from build123d import *

# Parameters (mm, degrees)
F4_R      = 3.75
F4_R_2    = 2
F9_DEPTH  = 1.2
F10_DEPTH = 3.7
F11_DEPTH = 3
F12_DEPTH = 2.5
F13_DEPTH = 8
F14_D     = 2.5
F14_DEPTH = 6.0511758158
F15_D     = 1.4
F15_DEPTH = 11.001


with BuildPart() as f8:
    # F3 (on Front) → F8 (revolve)
    with BuildSketch(Plane.XZ):
        with BuildLine():
            Line((0, 42.7), (0, 0))
            Line((0, 0), (-8.38e-08, -21.7723533995))
            Line((-8.38e-08, -21.7723533995), (0.7499999162, -21.7723533995))
            Line((0.7499999162, -21.7723533995), (1.9999999162, -19))
            Line((1.9999999162, -19), (1.9999999162, -1.2))
            Line((1.9999999162, -1.2), (3.7499999162, -1.2))
            Line((3.7499999162, -1.2), (3.7499999162, 0))
            Line((3.7499999162, 0), (11, 0))
            Line((11, 0), (11, 1.6))
            Line((11, 1.6), (4.5, 1.6))
            Line((4.5, 1.6), (4.5, 2.6))
            Line((4.5, 2.6), (11, 2.6))
            Line((11, 2.6), (11, 4.1))
            Line((11, 4.1), (4.5, 4.1))
            Line((4.5, 4.1), (4.5, 5.1))
            Line((4.5, 5.1), (11, 5.1))
            Line((11, 5.1), (11, 6.6))
            Line((11, 6.6), (4.5, 6.6))
            Line((4.5, 6.6), (4.5, 7.6))
            Line((4.5, 7.6), (11, 7.6))
            Line((11, 7.6), (11, 9.1))
            Line((11, 9.1), (4.5, 9.1))
            Line((4.5, 9.1), (4.5, 10.1))
            Line((4.5, 10.1), (11, 10.1))
            Line((11, 10.1), (11, 11.6))
            Line((11, 11.6), (4.5, 11.6))
            Line((4.5, 11.6), (4.5, 12.6))
            Line((4.5, 12.6), (11, 12.6))
            Line((11, 12.6), (11, 14.1))
            Line((11, 14.1), (4.5, 14.1))
            Line((4.5, 14.1), (4.5, 15.1))
            Line((4.5, 15.1), (11, 15.1))
            Line((11, 15.1), (11, 16.6))
            Line((11, 16.6), (4.5, 16.6))
            Line((4.5, 16.6), (4.5, 17.6))
            Line((4.5, 17.6), (11, 17.6))
            Line((11, 17.6), (11, 19.1))
            Line((11, 19.1), (4.5, 19.1))
            Line((4.5, 19.1), (4.5, 20.1))
            Line((4.5, 20.1), (11, 20.1))
            Line((11, 20.1), (11, 21.6))
            Line((11, 21.6), (4.5, 21.6))
            Line((4.5, 21.6), (4.5, 22.6))
            Line((4.5, 22.6), (11, 22.6))
            Line((11, 22.6), (11, 24.1))
            Line((11, 24.1), (4.5, 24.1))
            Line((4.5, 24.1), (4.5, 25.1))
            Line((4.5, 25.1), (11, 25.1))
            Line((11, 25.1), (11, 26.6))
            Line((11, 26.6), (4.5, 26.6))
            Line((4.5, 26.6), (4.5, 28.1))
            Line((4.5, 28.1), (7.95, 28.1))
            Line((7.95, 28.1), (7.95, 29.1))
            Line((7.95, 29.1), (4.5, 29.1))
            Line((4.5, 29.1), (4.5, 30.6))
            Line((4.5, 30.6), (7.95, 30.6))
            Line((7.95, 30.6), (7.95, 33.1))
            Line((7.95, 33.1), (5.75, 33.1))
            Line((5.75, 33.1), (5.75, 39.1))
            Line((5.75, 39.1), (7.95, 39.1))
            Line((7.95, 39.1), (7.95, 42.7))
            Line((7.95, 42.7), (3.9007244632, 42.7))
            ThreePointArc((3.9007244632, 42.7), (4.6078312444, 42.9928932188), (4.9007244632, 43.7))
            Line((4.9007244632, 43.7), (4.9007244632, 50.8))
            ThreePointArc((4.9007244632, 50.8), (4.6078312444, 51.5071067812), (3.9007244632, 51.8))
            Line((3.9007244632, 51.8), (2.400000114, 51.8))
            Line((2.400000114, 51.8), (2.400000114, 52.05))
            Line((2.400000114, 52.05), (4.9007244632, 52.05))
            Line((4.9007244632, 52.05), (4.9007244632, 53.3001758158))
            Line((4.9007244632, 53.3001758158), (0, 53.3001758158))
            Line((0, 53.3001758158), (0, 51.8))
            Line((0, 51.8), (0, 42.7))
        make_face()
    revolve(axis=Axis((0, 0, 21.35), (0, 0, 1)))

    # F4 (on Top) → F9 (join)
    with BuildSketch(Plane.XY):
        Circle(F4_R)
        Circle(F4_R_2, mode=Mode.SUBTRACT)
    extrude(amount=-F9_DEPTH)

    # F4 (on Top) → F10 (join)
    with BuildSketch(Plane.XY):
        Circle(F4_R_2)
    extrude(amount=-F10_DEPTH)

    # F5 (on offset) → F11 (join)
    with BuildSketch(Plane.XY.offset(-19)):
        Polygon((4.5, -2.5980762114), (4.5, 2.5980762114), (0, 5.1961524227), (-4.5, 2.5980762114), (-4.5, -2.5980762114), (0, -5.1961524227), align=None)
    extrude(amount=F11_DEPTH)

    # F6 (on offset) → F12 (join, symmetric)
    with BuildSketch(Plane.XY.offset(47.25)):
        Polygon((5, -2.8867513459), (5, 2.8867513459), (0, 5.7735026919), (-5, 2.8867513459), (-5, -2.8867513459), (0, -5.7735026919), align=None)
    extrude(amount=F12_DEPTH, both=True)

    # F7 (on Right) → F13 (join, symmetric)
    with BuildSketch(Plane.YZ):
        with BuildLine():
            Line((15.400047414, -3.6999706645), (-4.6000713482, -3.6999706645))
            Line((-4.6000713482, -3.6999706645), (-4.6000713482, -15.7000441104))
            Line((-4.6000713482, -15.7000441104), (15.400047414, -15.7000441104))
            Line((15.400047414, -15.7000441104), (15.400047414, -8.1999711692))
            Line((15.400047414, -8.1999711692), (9.8358729723, -8.1999711692))
            ThreePointArc((9.8358729723, -8.1999711692), (4.1714493177, -10.0637568305), (9.2873664374, -6.9999708794))
            Line((9.2873664374, -6.9999708794), (15.400047414, -6.9999708794))
            Line((15.400047414, -6.9999708794), (15.400047414, -3.6999706645))
        make_face()
    extrude(amount=F13_DEPTH, both=True)

    # F14 (through all, one way)
    with BuildSketch(Plane(origin=(0, 0, 47.25), x_dir=(1, 0, 0), z_dir=(0, 0, -1))):
        with Locations((0, 0)):
            Circle(F14_D / 2)
    extrude(amount=-F14_DEPTH, mode=Mode.SUBTRACT)

    # F15 (through all, one way)
    with BuildSketch(Plane(origin=(0, 0, 0), x_dir=(0, 1, 0), z_dir=(-1, 0, 0))):
        with Locations((-3.0674322043, 8.1999711692)):
            Circle(F15_D / 2)
    extrude(amount=-F15_DEPTH, mode=Mode.SUBTRACT)


solid = f8.part
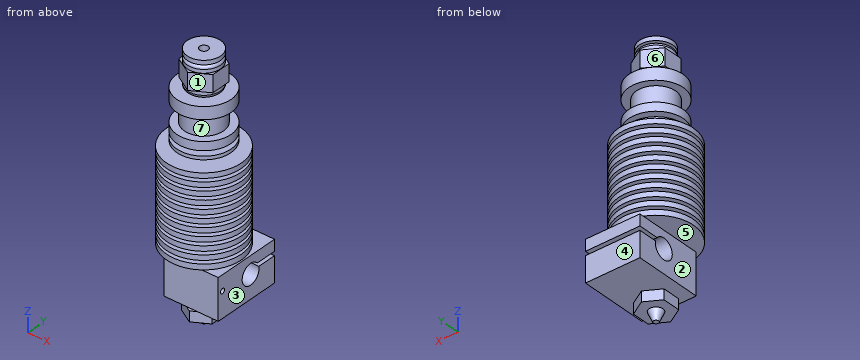
Input: part model. Units: mm. Frame: model coordinates. Face numbers are marked on the shaded views. A direction names the side the tool comes from. Round coordinates to 2 decimals unless told otherwise and drop trailing zeros. Order: outer loops, then holes, each group sorted by start corner. A loop starts at its lowest first (then second) coordinate and runs counter-clockwise, first axis right, second up.
1. Pin query (flat end, axial travel): P1, Ø10, axis at x = 7, y = 10.5, coming from the +Z side; P2, Ø1.3, axis at y = -3.07, z = -8.2, coming from the -X side; P3, Ø10, axis at x = 6, z = 5, coming from the -Y side. Return the tip coordinate at first contact, or that it passes through.
The answers:
P1: stops at z = 42.7
P2: stops at x = -8
P3: stops at y = -10.95
2. Cut plane A-A, the plane x = 7.25. State how many separate pieces and enclosed holes the cut face has, then the cut area to 3 significant figures.
The answers:
separate pieces: 15
enclosed holes: 1
area: 524 mm2
3. Mould query, pull axis Z, two halves, no side actions, for the marked faces 5, 6 and 7. Classes: released by +Z, released by -Z, zero draft, split by the parting line, or undercut.
The answers:
face 5: undercut
face 6: zero draft
face 7: undercut
4. Material intervals for line 1 (Y direction, x = 0, z = 49.25); line 2 (Z direction, x = -5.75, y = 12.75); line 3 (Y direction, x = 0, z = 52), sorted ascending.
The answers:
line 1: y = -5.77 to -1.25, 1.25 to 5.77
line 2: z = -15.7 to -8.2, -7 to -3.7
line 3: y = -2.4 to -1.25, 1.25 to 2.4
5. Cut plane C-C, the plane z = 41. Output: boundary loops of the cut face in (x, y).
The answers:
outline: circle Ø15.9 at (0, 0)
6. Set-up query: the marked faces 1, 2, 3 and 4. Return all of +Z, -Z, +X, -X, +Y, -Y with unobstructed straight access to the full face (end or side cutting, diameter ignored); none if empty.
The answers:
face 1: +Z, +X, -Y
face 2: -Z, -X, +Y, -Y
face 3: -Z, +X, +Y, -Y
face 4: +Z, -Z, +X, -X, +Y
